Input: part model. Units: mm. Frame: model coordinates. A direction names the side the tool comes from. Round coordinates to 2 decimals unless told otherwise and drop trailing zeros. Write each loop counter-clockwise with the first axis right and the second up, starting at its lowest first coordinate (ties: lowest second). Pieces come first, ordered by that corner, then holes. Notation, with made-up numbers: (86.25, -22) -> (124.25, -22) arc R36 ccw to (124.25, 16) -> close; hole circle Ø1 at (62, 4.5). An arc over 180 degrees is marked (long way). Write item = value, one per line. Start each with the question number.
```python
from build123d import *

# Parameters (mm, degrees)
BOSS_EXTRUDE1_DEPTH = 25
SHELL1_T            = -2
SKETCH4_R           = 5
CUT_EXTRUDE2_DEPTH  = 40
SKETCH5_R           = 5.211475532
BOSS_EXTRUDE2_DEPTH = 3
CUT_EXTRUDE3_DEPTH  = 53
BOSS_EXTRUDE3_DEPTH = 3
SKETCH8_R           = 4.596631542
CUT_EXTRUDE4_DEPTH  = 3
BOSS_EXTRUDE4_DEPTH = 3
CUT_EXTRUDE5_DEPTH  = 3
CUT_EXTRUDE6_DEPTH  = 3
CUT_EXTRUDE7_DEPTH  = 3
BOSS_EXTRUDE5_DEPTH = 3
SKETCH14_R          = 4.596631542
CUT_EXTRUDE8_DEPTH  = 23
CUT_EXTRUDE10_DEPTH = 23


with BuildPart() as part:
    # Sketch1 → Boss-Extrude1 (new body)
    with BuildSketch(Plane(origin=(0, 0, 0), x_dir=(1, 0, 0), z_dir=(0, 1, 0))):
        Polygon((125.56624327, 217.48711306), (-125.56624327, 217.48711306), (-251.132486541, 0), (-125.56624327, -217.48711306), (125.56624327, -217.48711306), (251.132486541, 0), (280, 0), (140, -242.48711306), (-140, -242.48711306), (-280, 0), (-140, 242.48711306), (140, 242.48711306), align=None)
    extrude(amount=BOSS_EXTRUDE1_DEPTH)

    # Shell1
    shell1_openings = [part.faces().sort_by_distance(p)[0] for p in [
        (265.56624327, 12.5, 0),
        (132.783121635, 12.5, -229.98711306),
    ]]
    offset(amount=SHELL1_T, openings=shell1_openings, kind=Kind.INTERSECTION)

    # Sketch4 → Cut-Extrude2 (cut)
    with BuildSketch(Plane(origin=(0, 25, 0), x_dir=(1, 0, 0), z_dir=(0, 1, 0))):
        with Locations((180.587500524, -147.1875)):
            Circle(SKETCH4_R)
    extrude(amount=-CUT_EXTRUDE2_DEPTH, mode=Mode.SUBTRACT)

    # Sketch5 → Boss-Extrude2 (add)
    with BuildSketch(Plane(origin=(0, 25, 0), x_dir=(1, 0, 0), z_dir=(0, 1, 0))):
        Polygon((201.132486541, -86.602540378), (159.222437422, -159.192874799), (98.600659157, -124.192874799), (140.510708276, -51.602540378), align=None)
        with Locations((121.228675973, -125)):
            Circle(SKETCH5_R, mode=Mode.SUBTRACT)
    extrude(amount=-BOSS_EXTRUDE2_DEPTH)

    # Sketch6 → Cut-Extrude3 (cut)
    with BuildSketch(Plane(origin=(0, 25, 0), x_dir=(1, 0, 0), z_dir=(0, 1, 0))):
        Polygon((140.510708276, -51.602540378), (201.132486541, -86.602540378), (158.682929972, -160.127329114), (98.061151707, -125.127329114), align=None)
    extrude(amount=-CUT_EXTRUDE3_DEPTH, mode=Mode.SUBTRACT)

    # Sketch7 → Boss-Extrude3 (add)
    with BuildSketch(Plane(origin=(0, 25, 0), x_dir=(1, 0, 0), z_dir=(0, 1, 0))):
        Polygon((227.297559203, -41.283305143), (205.297559203, -79.388422909), (149.005907957, -46.888422909), (171.005907957, -8.783305143), align=None)
    extrude(amount=-BOSS_EXTRUDE3_DEPTH)

    # Sketch8 → Cut-Extrude4 (cut)
    with BuildSketch(Plane(origin=(0, 25, 0), x_dir=(1, 0, 0), z_dir=(0, 1, 0))):
        with Locations((196.32303906, -78.932747771)):
            Circle(SKETCH8_R)
    extrude(amount=-CUT_EXTRUDE4_DEPTH, mode=Mode.SUBTRACT)

    # Sketch9 → Boss-Extrude4 (add)
    with BuildSketch(Plane(origin=(0, 25, 0), x_dir=(1, 0, 0), z_dir=(0, 1, 0))):
        with BuildLine():
            Line((205.297559203, -79.388422909), (200.181682496, -76.434770115))
            ThreePointArc((200.181682496, -76.434770115), (194.024723289, -82.913547458), (196.55702945, -74.342075704))
            Line((196.55702945, -74.342075704), (149.005907957, -46.888422909))
            Line((149.005907957, -46.888422909), (138.101240513, -65.775860963))
            Line((138.101240513, -65.775860963), (194.392891759, -98.275860963))
            Line((194.392891759, -98.275860963), (205.297559203, -79.388422909))
        make_face()
    extrude(amount=-BOSS_EXTRUDE4_DEPTH)

    # Sketch10 → Cut-Extrude5 (cut)
    with BuildSketch(Plane(origin=(0, 25, 0), x_dir=(1, 0, 0), z_dir=(0, 1, 0))):
        Polygon((171.005907957, -8.783305143), (227.297559203, -41.283305143), (211.247303055, -69.083164267), (154.955651809, -36.583164267), align=None)
    extrude(amount=-CUT_EXTRUDE5_DEPTH, mode=Mode.SUBTRACT)

    # Sketch11 → Cut-Extrude6 (cut)
    with BuildSketch(Plane(origin=(0, 25, 0), x_dir=(1, 0, 0), z_dir=(0, 1, 0))):
        Polygon((154.955651809, -36.583164267), (189.376099165, -56.455818813), (172.628994903, -85.462654274), (138.208547547, -65.589999728), align=None)
    extrude(amount=-CUT_EXTRUDE6_DEPTH, mode=Mode.SUBTRACT)

    # Sketch12 → Cut-Extrude7 (cut)
    with BuildSketch(Plane(origin=(0, 25, 0), x_dir=(1, 0, 0), z_dir=(0, 1, 0))):
        Polygon((133.472959546, -64.327583033), (137.505827692, -57.317833183), (175.943359627, -79.431817482), (171.910491481, -86.441567333), align=None)
    extrude(amount=-CUT_EXTRUDE7_DEPTH, mode=Mode.SUBTRACT)

    # Sketch13 → Boss-Extrude5 (add)
    with BuildSketch(Plane.XZ):
        Polygon((197.947448943, 92.119187322), (189.768280461, 106.285922696), (211.418915556, 118.785922696), (235.385066588, 77.275331446), (213.403041068, 64.584003094), (211.247303055, 69.083164267), (189.376099165, 56.455818813), (176.035335717, 79.351557189), align=None)
    extrude(amount=BOSS_EXTRUDE5_DEPTH)

    # Sketch14 → Cut-Extrude8 (cut)
    with BuildSketch(Plane(origin=(0, 0, 0), x_dir=(1, 0, 0), z_dir=(0, 1, 0))):
        with Locations((192.705001821, -81.222810357)):
            Circle(SKETCH14_R)
    extrude(amount=-CUT_EXTRUDE8_DEPTH, mode=Mode.SUBTRACT)

    # Sketch15 → Cut-Extrude10 (cut)
    with BuildSketch(Plane(origin=(0, 25, 0), x_dir=(1, 0, 0), z_dir=(0, 1, 0))):
        Polygon((187.452678382, -55.345331307), (211.247303055, -69.083164267), (194.392891759, -98.275860963), (170.321525229, -84.378251017), align=None)
    extrude(amount=-CUT_EXTRUDE10_DEPTH, mode=Mode.SUBTRACT)


solid = part.part
```
1. Section B-B (z = 159). Output: boundary loops of the cut face in (x, y), then the cut area to 3 significant figures.
2. Line query: line 1 along Z through (x, y) = (-37.5, 4.5); line 2 along Z through (x, y) = (-203, 13); line 3 along X through (y, z) = (13.75, 182). Output: solid intervals per line, ascending.
3. Reachability of faces 5 (the flat face through (2, 12, -219.487)), 6 (the flat face through (-204, 2, 88)), 7 (the flat face through (-187.47, 12.32, -110.27)), 8 (the flat face through (200.465, -1.479, 62.858)) from +Z, -Z, +X, -X, +Y, -Y: full face, straight path, thin tool, end or side. Return the list, or none.
4. Section D-D (z = -44.5). Output: boundary loops of the cut face in (x, y), then the cut area to 3 significant figures.
5. Pin query (flat end, axial travel): P1, Ø5, axis at x = -196, y = 7.5, coming from the -Z side; P2, Ø12, axis at y = 1, z = 49, coming from the -X side; P3, Ø7.5, axis at x = 268.5, y = 18, coming from the -Z side; P4, Ø5.5, axis at x = 192.71, z = 81.22, coming from the +Y side. Return the tip coordinate at first contact, or that it passes through.
6. Section A-A (x = -12). Output: boundary loops of the cut face in (y, z), then the cut area to 3 significant figures.
7. Section C-C (y = 16.5). Output: boundary loops of the cut face in (x, z), then the cut area to 3 significant figures.
8. Mould query, pull axis Z, two halves, no side actions, for faces 1 (the flat face through (209.24, 12.35, 118.56)), 2 (the flat face through (-189.23, 12.32, 107.22)), 3 (the flat face through (206, -3, 88)), 4 (the flat face through (-2, 12, -242.487)). Classes: pulls with the +Z half, pulls with the -Z half, needs draft (parallel to the pull), parting line crosses it, or undercut.
Check sheet entries:
q1.outline = (-188.2, 0) -> (-159.33, 0) -> (-159.33, 25) -> (-188.2, 25) -> close; (159.33, 0) -> (188.2, 0) -> (188.2, 25) -> (159.33, 25) -> close; hole (-185.89, 2) -> (-161.64, 2) -> (-161.64, 23) -> (-185.89, 23) -> close; hole (161.64, 2) -> (185.89, 2) -> (185.89, 23) -> (161.64, 23) -> close
q1.area = 425 mm2
q2.line_1 = -242.49 to -240.49, -219.49 to -217.49, 217.49 to 219.49, 240.49 to 242.49
q2.line_2 = -133.37 to -129.37, -87.37 to -83.37, 83.37 to 87.37, 129.37 to 133.37
q2.line_3 = -174.92 to -172.61, -148.36 to -146.05, 146.05 to 148.36, 172.61 to 174.92
q3.face_5 = +X
q3.face_6 = none
q3.face_7 = +X, +Y, -Y
q3.face_8 = -Z, +Y, -Y
q4.outline = (-254.31, 0) -> (-225.44, 0) -> (-225.44, 25) -> (-254.31, 25) -> close; hole (-252, 2) -> (-227.75, 2) -> (-227.75, 23) -> (-252, 23) -> close
q4.area = 212 mm2
q5.P1 = -149.82
q5.P2 = -255.17
q5.P3 = 9.42
q5.P4 = through
q6.outline = (0, -242.49) -> (25, -242.49) -> (25, -217.49) -> (0, -217.49) -> close; (0, 217.49) -> (25, 217.49) -> (25, 242.49) -> (0, 242.49) -> close; hole (2, -240.49) -> (23, -240.49) -> (23, -219.49) -> (2, -219.49) -> close; hole (2, 219.49) -> (23, 219.49) -> (23, 240.49) -> (2, 240.49) -> close
q6.area = 368 mm2
q7.outline = (-280, 0) -> (-140, -242.49) -> (140, -242.49) -> (138.85, -240.49) -> (-138.85, -240.49) -> (-277.69, 0) -> (-138.85, 240.49) -> (138.85, 240.49) -> (277.69, 0) -> (280, 0) -> (140, 242.49) -> (-140, 242.49) -> close; (-253.44, 0) -> (-126.72, -219.49) -> (126.72, -219.49) -> (125.57, -217.49) -> (-125.57, -217.49) -> (-251.13, 0) -> (-125.57, 217.49) -> (125.57, 217.49) -> (251.13, 0) -> (253.44, 0) -> (126.72, 219.49) -> (-126.72, 219.49) -> close
q7.area = 5,310 mm2
q8.face_1 = undercut
q8.face_2 = undercut
q8.face_3 = needs draft
q8.face_4 = pulls with the -Z half
